Verification items for the finished model (mm, model axes). Face numbers are marked on the shaded views. A direction names the side the tool comes from. Give positions to 0.01 mm unless a question says otherwise; leave off trailing zeros. Order: outer loops, then holes, each group sorted by start corner. A loop starts at its lowest first (then second) coordinate and runs counter-clockwise, first axis right, second up. Notation, with made-up numbers: (80.25, -30) -> (98.25, -30) arc R22 cw to (98.25, -16) -> close; hole circle Ø11 at (-15, 28.25). An arc over 180 degrees is marked (long way). Return JSON: item names as keys, results as strings. Group by question number.
(1) Cross-section at D-D on y = -1.5. Enter the section's corners in (x, z).
(2) Thickness scan on line 1 along X through (y, z) = (29, 5); line 2 along Y through (x, z) = (6.5, 24); line 3 along Y through (x, z) = (4.75, -2.5). Record the ranges inside material, lowest first.
(3) Depth check by flat-ended pin: pin 1 Ø6 at (x, y) = (-7, 6.5) entering from +Z; pin 2 Ø12 at (y, z) = (20.5, 12.5) entering from -X; pin 3 Ø1.5 at (x, y) = (-7, 0.5) entering from -Z. Enter the tip coordinate at first touch or a pass-through.
(4) Cross-section at C-C on y = 10.5. Enter the section's corners in (x, z).
(5) Cross-section at A-A on z = 20. Enter the section's corners in (x, y).
(6) Tool access check on the marked faces 1, 2, 3 and 4. Record the directions out of +Z, -Z, +X, -X, +Y, -Y that give a thin tool (end or side, any length) a straight path to the whole face; none if there is none.
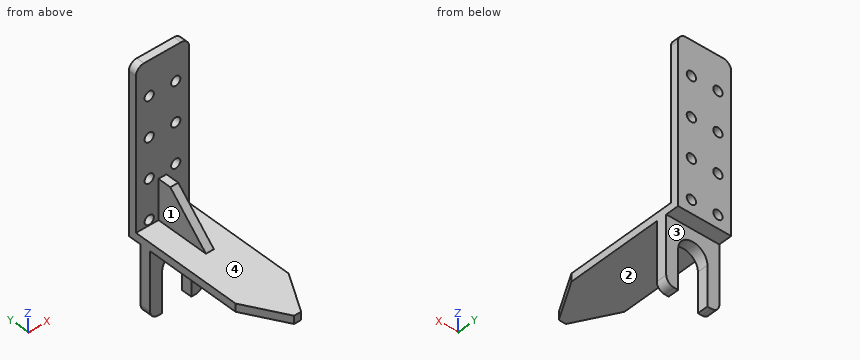
from build123d import *
from OCP.BRepFilletAPI import BRepFilletAPI_MakeChamfer

# Parameters (mm, degrees)
SKETCH1_W           = 20
SKETCH1_H           = 60
BOSS_EXTRUDE1_DEPTH = 3
SKETCH2_W           = 20
SKETCH2_H           = 3
BOSS_EXTRUDE2_DEPTH = 60
SKETCH3_W           = 3
SKETCH3_H           = 15
BOSS_EXTRUDE3_DEPTH = 20
CHAMFER1_SIZE       = 15
SKETCH4_R           = 1.75
CUT_EXTRUDE1_DEPTH  = 86.545309632
LPATTERN1_COUNT     = 4
LPATTERN1_PITCH     = 15
CHAMFER2_SIZE       = 15
CHAMFER2_SIZE2      = 8.660254038
FILLET1_R           = 3
SKETCH5_W           = 20
SKETCH5_H           = 4
BOSS_EXTRUDE4_DEPTH = 25
CUT_EXTRUDE2_DEPTH  = 85.225886757
FILLET2_R           = 3


with BuildPart() as part:
    # Sketch1 → Boss-Extrude1 (new body)
    with BuildSketch(Plane.XY):
        Rectangle(SKETCH1_W, SKETCH1_H)
    extrude(amount=BOSS_EXTRUDE1_DEPTH)

    # Sketch2 → Boss-Extrude2 (add)
    with BuildSketch(Plane.XY.offset(3)):
        with Locations((0, 28.5)):
            Rectangle(SKETCH2_W, SKETCH2_H)
    extrude(amount=BOSS_EXTRUDE2_DEPTH)

    # Sketch3 → Boss-Extrude3 (add)
    with BuildSketch(Plane.XZ.offset(-27)):
        with Locations((0, 10.5)):
            Rectangle(SKETCH3_W, SKETCH3_H)
    extrude(amount=BOSS_EXTRUDE3_DEPTH)

    # Chamfer1
    chamfer1_edges = [part.edges().sort_by_distance(p)[0] for p in [
        (0, 7, 18),
    ]]
    chamfer(chamfer1_edges, length=CHAMFER1_SIZE - 0.0001)  # a hair under: the kernel refuses the full size

    # Sketch4 → Cut-Extrude1 (cut, through all)
    with BuildSketch(Plane.XZ.offset(-27)):
        with Locations(Location((-5, 5, 0), (0, 0, 270))):
            Circle(SKETCH4_R)
        with Locations(Location((5, 5, 0), (0, 0, 270))):
            Circle(SKETCH4_R)
    cut_extrude1 = extrude(amount=-CUT_EXTRUDE1_DEPTH, mode=Mode.SUBTRACT)

    # LPattern1: Cut-Extrude1 ×4
    with Locations(*[(0, 0, i * LPATTERN1_PITCH) for i in range(1, LPATTERN1_COUNT)]):
        add(cut_extrude1, mode=Mode.SUBTRACT)

    # Chamfer2: one chamfer whose edges measure the first distance from different faces: ONE call of the kernel's chamfer builder (chamfer() names one face for all edges)
    chamfer2_edges_1 = [part.edges().sort_by_distance(p)[0] for p in [
        (10, -30, 1.5),
    ]]
    chamfer2_side_1 = [part.faces().sort_by_distance(p)[0] for p in [
        (10, 29.13, 31.5),
    ]]
    chamfer2_edges_2 = [part.edges().sort_by_distance(p)[0] for p in [
        (-10, -30, 1.5),
    ]]
    chamfer2_side_2 = [part.faces().sort_by_distance(p)[0] for p in [
        (-10, -29.13, 1.5),
    ]]
    chamfer2 = BRepFilletAPI_MakeChamfer(part.part.solid().wrapped)
    for e in chamfer2_edges_1:
        chamfer2.Add(CHAMFER2_SIZE, CHAMFER2_SIZE2, e.wrapped, chamfer2_side_1[0].wrapped)  # the first distance lies on this face
    for e in chamfer2_edges_2:
        chamfer2.Add(CHAMFER2_SIZE, CHAMFER2_SIZE2, e.wrapped, chamfer2_side_2[0].wrapped)  # the first distance lies on this face
    add(Compound.cast(chamfer2.Shape()), mode=Mode.REPLACE)

    # Fillet1
    fillet1_edges = [part.edges().sort_by_distance(p)[0] for p in [
        (-10, 28.5, 63),
        (10, 28.5, 63),
    ]]
    fillet(fillet1_edges, radius=FILLET1_R)

    # Sketch5 → Boss-Extrude4 (add)
    with BuildSketch(Plane(origin=(0, 0, 0), x_dir=(-1, 0, 0), z_dir=(0, 0, -1))):
        with Locations((0, 23)):
            Rectangle(SKETCH5_W, SKETCH5_H)
    extrude(amount=BOSS_EXTRUDE4_DEPTH)

    # Sketch6 → Cut-Extrude2 (cut, through all)
    with BuildSketch(Plane(origin=(0, 25, 0), x_dir=(1, 0, 0), z_dir=(0, 1, 0))):
        with BuildLine():
            Line((-5.5, 10), (-5.5, 25))
            Line((-5.5, 25), (5.5, 25))
            Line((5.5, 25), (5.5, 10))
            ThreePointArc((5.5, 10), (0, 4.5), (-5.5, 10))
        make_face()
    extrude(amount=-CUT_EXTRUDE2_DEPTH, mode=Mode.SUBTRACT)

    # Fillet2
    fillet2_edges = [part.edges().sort_by_distance(p)[0] for p in [
        (10, 23, -25),
        (-10, 23, -25),
    ]]
    fillet(fillet2_edges, radius=FILLET2_R)


solid = part.part
Verdict:
{
 "1": {"outline": "(-10, 0) -> (10, 0) -> (10, 3) -> (-10, 3) -> close"},
 "2": {"line 1": "-10 to -6.75, -3.25 to 3.25, 6.75 to 10", "line 2": "27 to 30", "line 3": "21 to 25"},
 "3": {"pin 1": "z = 3", "pin 2": "x = -1.5", "pin 3": "z = 0"},
 "4": {"outline": "(-10, 0) -> (10, 0) -> (10, 3) -> (1.5, 3) -> (1.5, 6.5) -> (-1.5, 6.5) -> (-1.5, 3) -> (-10, 3) -> close"},
 "5": {"outline": "(-10, 27) -> (-6.75, 27) -> (-6.75, 30) -> (-10, 30) -> close; (-3.25, 27) -> (3.25, 27) -> (3.25, 30) -> (-3.25, 30) -> close; (6.75, 27) -> (10, 27) -> (10, 30) -> (6.75, 30) -> close"},
 "6": {"face 1": "+Z, -X, -Y", "face 2": "-Z, +X, -X, -Y", "face 3": "-Z, +X, -X, +Y", "face 4": "+Z, -Y"}
}
